Geometry check sheet. Reference: the model listing, model coordinates, mm. A direction names the side the tool comes from. Round coordinates to 2 decimals unless told otherwise and drop trailing zeros. Order: outer loops, then holes, each group sorted by start corner. A loop starts at its lowest first (then second) coordinate and runs counter-clockwise, first axis right, second up. Notation, with made-up numbers: (12.5, -15.5) - (68.5, -15.5) arc R23 ccw to (68.5, 17.5) - close; hole circle Ø7 at (-34.75, 27.5). An arc over 180 degrees is marked (long way). Write each question's results on one line, items separated by ' | '.
Autodesk Inventor part; units mm, degrees
ref_plane "YZ Plane" through (0, 0, 0) normal (1, 0, 0) x (0, 1, 0)
ref_plane "XZ Plane" through (0, 0, 0) normal (0, 1, 0) x (-1, 0, 0)
ref_plane "XY Plane" through (0, 0, 0) normal (0, 0, 1) x (1, 0, 0)
sketch "Sketch1" plane through (0, 0, 0) normal (0, 0, 1) x (1, 0, 0)
  line L0 (-490, 68) -> (490, 68)
  line L1 (490, 68) -> (490, 0)
  line L2 (490, 0) -> (-490, 0)
  line L3 (-490, 0) -> (-490, 68)
  point P0 (0, 0)
  point P1 (0, 0)
  dimension "d0" = 980
  dimension "d1" = 68
extrude "Plate1" add sketch "Sketch1" along normal blind 2
sketch "Sketch2" plane through (490, 2, 0) normal (0, -1, 0) x (1, 0, 0)
  line L0 (-980, 0) -> (0, 0)
  line L1 (0, 0) -> (0, 20)
  line L2 (0, 20) -> (-980, 20)
  line L3 (-980, 20) -> (-980, 0)
edge flange "Flange1" height 20 angle 90 thickness 2 bend radius 2.75 thickness toward (0, -1, 0) relief round relief width 2 relief depth 1 edges at (0, 0, 2) wall of the first edge with corners at (-490, 2, 0) (490, 2, 0) (490, 2, 20) (-490, 2, 20)
bend "Bend1"
corner "Corner1"
sketch "Sketch5" plane through (0, 0, 0) normal (0, 0, -1) x (-1, 0, 0)
  line L0 (490, 68) -> (-490, 68)
  line L1 (490, 0) -> (-490, 0)
  circle A0 centre (0, 68) radius 35
  line L2 (243.95, 68) -> (246.05, 68)
  line L3 (246.05, 68) -> (246.05, 29)
  line L4 (246.05, 29) -> (243.95, 29)
  line L5 (243.95, 29) -> (243.95, 68)
  line L6 (-243.95, 68) -> (-246.05, 68)
  line L7 (-246.05, 68) -> (-246.05, 29)
  line L8 (-246.05, 29) -> (-243.95, 29)
  line L9 (-243.95, 29) -> (-243.95, 68)
  line L10 (0, 68) -> (0, 0) construction
  line L11 (0, 68) -> (0, 0)
  line L12 (490, 68) -> (490, 4.75)
  line L13 (490, 0) -> (490, 4.75)
  line L14 (-490, 4.75) -> (-490, 68)
  line L15 (-490, 4.75) -> (-490, 0)
  point P0 (0, 0)
  point P1 (245, 29)
  point P2 (-245, 29)
  point P3 (-35, 68)
  point P4 (35, 68)
  dimension "d45" = 70
  dimension "d48" = 2.1
  dimension "d49" = 490
  dimension "d51" = 29
  dimension "d52" = 39
extrude "Extrusion1" cut sketch "Sketch5" against normal through all contours L12 L13 L1 L11 A0 L0 L5 L4 L3 | L3 L4 L5 L0 | A0 L11 L0 | L9 L8 L7 L0 picked at (23.0408, 65.4039)
sketch "Sketch9" plane through (0, 0, 2) normal (0, 0, 1) x (1, 0, 0)
  line L0 (485.6141, 29.596) -> (485.6141, 17.596) construction
  line L1 (485.6141, 17.596) -> (285.6141, 17.596) construction
  line L2 (285.6141, 17.596) -> (285.6141, 29.596) construction
  line L3 (285.6141, 29.596) -> (485.6141, 29.596) construction
  line L4 (-490, 68) -> (490, 68)
  point P0 (0, 0)
  point P1 (1.05, 68)
  dimension "d40" = 200
  dimension "d41" = 12
mark "Mark2"
equation "\"d1\" = СПИНА_Стрингер_2_высота"
equation "\"d2\" = Thickness"
equation "\"d3\" = BendReliefWidth"
equation "\"d4\" = BendReliefDepth"
equation "\"d5\" = MinimumRemnant"
equation "\"d6\" = TransitionRadius"
equation "\"d9\" = BendRadius"
equation "\"d10\" = CornerReliefSize"
equation "\"d11\" = GapSize"
equation "\"d12\" = JacobiRadiusSize"
equation "\"BendReliefWidth\" = Thickness"
equation "\"BendReliefDepth\" = 0.5 * Thickness"
equation "\"CornerReliefSize\" = 4 * Thickness"
equation "\"MinimumRemnant\" = 2 * Thickness"
equation "\"TransitionRadius\" = BendRadius"
equation "\"JacobiRadiusSize\" = BendRadius"
equation "\"GapSize\" = Thickness"
properties part number "MSC 207 stringer back ^^" material "Stainless Steel"
(1) Section check B-B (x = 188). Record the cut outline in (y, z), then the cut area to 3 significant figures.
Answers follow:
outline: (0, 4.75) arc R4.75 ccw to (4.75, 0) - (68, 0) - (68, 2) - (4.75, 2) arc R2.75 cw to (2, 4.75) - (2, 20) - (0, 20) - close | area: 169 mm²
(2) Material ranges on line 1 (X direction, y = 31.5, z = 1.5); line 2 (Y direction, x = 234.5, z = 18.5), recorded low to high.
Answers follow:
line 1: 0 to 243.95, 246.05 to 490 | line 2: 0 to 2
(3) Section check A-A (y = 56.5). Record the cut outline in (x, z).
Answers follow:
outline: (0, 0) - (243.95, 0) - (243.95, 2) - (0, 2) - close; (246.05, 0) - (490, 0) - (490, 2) - (246.05, 2) - close
(4) Depth check by flat-ended pin: pin 1 Ø4 at (x, z) = (234, 11) entering from +Y; pin 2 Ø12 at (x, z) = (251, 8.5) entering from +Y; pin 3 Ø1 at (x, z) = (245, 0.5) entering from +Y. Enter the tip coordinate at first touch or a pass-through.
Answers follow:
pin 1: y = 2 | pin 2: y = 3.17 | pin 3: y = 29
(5) Section check C-C (z = 13.5). Record the cut outline in (x, y), then the cut area to 3 significant figures.
Answers follow:
outline: (0, 0) - (490, 0) - (490, 2) - (0, 2) - close | area: 980 mm²
(6) Access from +Z, -Z, +X, -X, +Y, -Y to the whole of each face (thin tool, end or side, straight path). Record for faces 1 (the face through (242, 37, 0)), 2 (the face through (242, 37, 2)).
Answers follow:
face 1: -Z, +X, -X, +Y, -Y | face 2: +Z, +X, -X, +Y
